Can you work these out from the model? Positions are in its coordinate system, mm. Face numbers are marked on the shaded views. Coordinates: 2 decimals unless noted, no trailing zeros. Order: outer loops, then holes, each group sorted by start corner. A loop starts at its lowest first (then second) coordinate and runs counter-clockwise, first axis right, second up.
```python
from build123d import *

# Parameters (mm, degrees)
F1_START = 3
F0_R     = 31
F0_R_2   = 27.5
F1_DEPTH = 66
F0_R_3   = 9
F2_DEPTH = 72


with BuildPart() as f1:
    # F0 (on Top) → F1 (new body)
    with BuildSketch(Plane.XY.offset(F1_START)):
        Circle(F0_R)
        Circle(F0_R_2, mode=Mode.SUBTRACT)
    extrude(amount=F1_DEPTH)

    # F0 (on Top) → F2 (join)
    with BuildSketch(Plane.XY):
        Circle(F0_R_2)
        Circle(F0_R_3, mode=Mode.SUBTRACT)
    extrude(amount=F2_DEPTH)


solid = f1.part
```
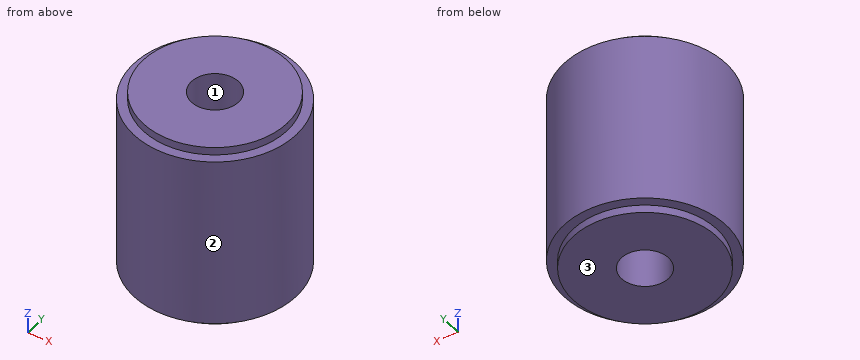
1. Imagine slicing it at A-A on y = 0. Please give me the cut outline in (x, z).
Completed:
outline: (-31, 3) - (-27.5, 3) - (-27.5, 0) - (-9, 0) - (-9, 72) - (-27.5, 72) - (-27.5, 69) - (-31, 69) - close; (9, 0) - (27.5, 0) - (27.5, 3) - (31, 3) - (31, 69) - (27.5, 69) - (27.5, 72) - (9, 72) - close
2. I'm going to push flat-ended pins straight in: pin 1 (6 mm diameter, centred on y = 12.5, z = 35.5, fed in from -X); pin 2 (6 mm diameter, centred on y = -19, z = 36.5, fed in from -X); pin 3 (1.5 mm diameter, centred on x = 21, z = 40, fed in from +Y); pin 4 (20.5 mm diameter, centred on x = 0, y = 0, fed in from -Z). Where does each tip first touch, or does it pass through?
Completed:
pin 1: stops at x = -29.51
pin 2: stops at x = -26.55
pin 3: stops at y = 23.47
pin 4: stops at z = 0
3. Thinking about a two-plate mould opening in X: for the marked faces 1, 2 and 3, which applies, pulls with the +X half, pulls with the -X half, needs draft (parallel to the pull), parting line crosses it, or undercut?
Completed:
face 1: undercut
face 2: parting line crosses it
face 3: needs draft
4. Please list where these lines run through material, in increasing order: probe 1 along Y at (x, z) = (0, 18); probe 2 along X at (y, z) = (-5, 54.5); probe 3 along Z at (x, y) = (-8, 27).
Completed:
probe 1: y = -31 to -9, 9 to 31
probe 2: x = -30.59 to -7.48, 7.48 to 30.59
probe 3: z = 3 to 69
5. Imagine slicing it at D-D on x = -11. Please give me the cut outline in (y, z), then the cut area to 3 significant figures.
Completed:
outline: (-28.98, 3) - (-25.2, 3) - (-25.2, 0) - (25.2, 0) - (25.2, 3) - (28.98, 3) - (28.98, 69) - (25.2, 69) - (25.2, 72) - (-25.2, 72) - (-25.2, 69) - (-28.98, 69) - close
area: 4,130 mm2
6. Imagine slicing it at C-C on z = 62. Please give me the cut outline in (x, y).
Completed:
outline: circle Ø62 at (0, 0); hole circle Ø18 at (0, 0)
